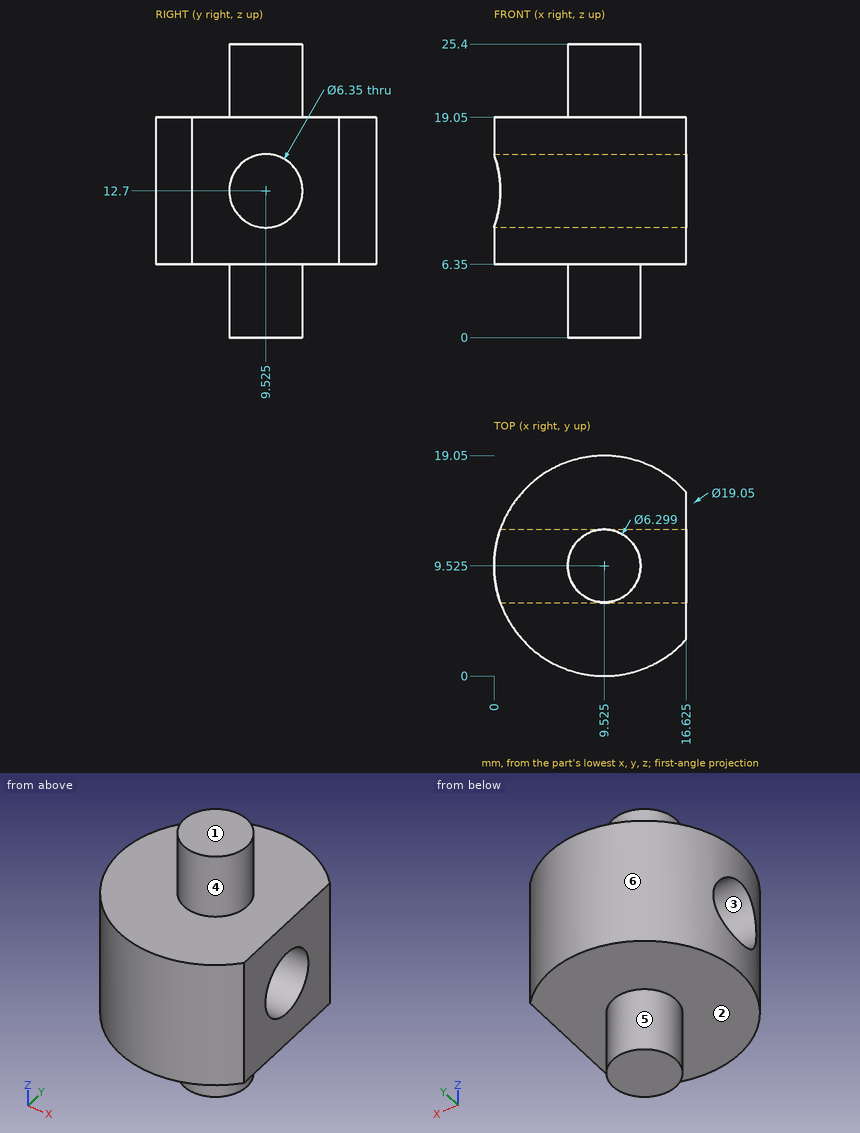
Geometry: see drawing. Coordinates: mm, zero at the bounding-box minimum. A direction names the side the tool comes from. Round coordinates to 2 decimals unless told otherwise and drop trailing zeros.
1) Ray query, L1, parallel to Y at x = 9.75, z = 12.7; L2, parallel to Z at x = 5, y = 1.25; L3, parallel to Y at x = 9.5, z = 2.25 (1 decimal). Return the intervals inside material, ascending.
2) Draft query along Z for the marked faces 1, 2 and 3. Return one class per face: pulls with the +Z half, pulls with the -Z half, needs draft (parallel to the pull), parting line crosses it, or undercut.
3) Contact query for flat-ended pins moving along their axis: P1, Ø4, axis at x = 4.5, z = 6, coming from the +Y side; P2, Ø5, axis at x = 3, y = 14, coming from the -Z side; P3, Ø3, axis at y = 2, z = 17.5, coming from the -X side; P4, Ø4, axis at y = 9.525, z = 12.7, coming from the -X side. Output: stop coordinate, or through.
4) Reachability of the marked faces 4, 5 and 6 from +Z, -Z, +X, -X, +Y, -Y: full face, straight path, thin tool, end or side. Return the list, or none.
Geometry says:
1. L1: y = 0 to 6.35, 12.7 to 19.05
1. L2: z = 6.35 to 19.05
1. L3: y = 6.4 to 12.7
2. face 1: pulls with the +Z half
2. face 2: pulls with the -Z half
2. face 3: undercut
3. P1: stops at y = 18.55
3. P2: stops at z = 6.35
3. P3: stops at x = 2.15
3. P4: passes through
4. face 4: +Z
4. face 5: -Z
4. face 6: +Z, -Z
